Design review of the part built by this model. Coordinates are the model's own, in mm. A direction names the side the tool comes from. Round coordinates to 2 decimals unless told otherwise and drop trailing zeros. Order: outer loops, then holes, each group sorted by start corner. A loop starts at its lowest first (then second) coordinate and runs counter-clockwise, first axis right, second up. Notation, with made-up numbers: M 21,46 L 33,46 A27 ccw 33,68 Z; hole C 68,-40 d6. An arc over 180 degrees is marked long. Use a Markdown table: item, result. Add a question column.
(1) Take a section at C-C (z = -11). Write out the cut boundary in (x, y), then the cut area to 3 significant figures.
(2) Machinability: for faces 5 (the face through (2.36, 5.87, 21.9)), 6 (the face through (4.483, 2.532, -23.147)), 7 (the face through (2.4, 5.87, -21.86)), which of the approach directions +Z, -Z, +X, -X, +Y, -Y give a long, thin tool a straight path to every point of the face, cutting with its end or side? Answer none if there is none.
(3) The part is to be moulded in two halves that separate along Y. For faces 1 (the face through (0, 0, 6)), 2 (the face through (8, 5.5, 24)), 3 (the face through (10.55, 2.58, 18.9)), 4 (the face through (-7.83, 1.97, 6.53)), say which applies: released by +Y, released by -Y, zero draft, split by the parting line, or undercut.
(4) To check wall thickness, follow probe 1 along X at (y, z) = (2.75, -21.75); probe 2 along Z at (x, y) = (-5, 5); probe 3 along Z at (x, y) = (0, 0.95). State the ranges of each line that lie inside material, in increasing order. Write a range as from..to.
(5) For pin 1 (1.8 mm diameter, centred on x = -3.5, y = 2.75, fed in from +Z); pin 2 (1.5 mm diameter, centred on x = 0, z = -11, fed in from -Y); pin 3 (4 mm diameter, centred on x = -10, z = 2, fed in from +Y), all flat-tipped, find the tip position at first contact; note any pin that passes through.
(6) Take a section at A-A (x = 0). Write out the cut boundary in (y, z).
(7) Take a section at B-B (y = 4.5). Write out the cut boundary in (x, z), then the cut area to 3 significant figures.
(8) Take a section at D-D (z = 22). Write out the cut boundary in (x, y).
Autodesk Inventor part; units mm, degrees
ref_plane "YZ Plane" through (0, 0, 0) normal (1, 0, 0) x (0, 1, 0)
ref_plane "XZ Plane" through (0, 0, 0) normal (0, 1, 0) x (-1, 0, 0)
ref_plane "XY Plane" through (0, 0, 0) normal (0, 0, 1) x (1, 0, 0)
sketch "Sketch1" plane through (0, 0, 0) normal (0, 1, 0) x (-1, 0, 0)
  line L0 (15, 27) -> (-15, 27)
  line L1 (-15, 27) -> (-15, -27)
  line L2 (-15, -27) -> (15, -27)
  line L3 (15, -27) -> (15, 27)
  line L4 (0, 27) -> (0, -27) construction
  line L5 (15, 0) -> (-15, 0) construction
  point P0 (0, 0)
  point P1 (0, 0)
  point P2 (15, 0)
  dimension "d0" = 54
  dimension "d1" = 30
extrude "Extrusion1" add sketch "Sketch1" along normal blind 6.25
sketch "Sketch2" plane through (0, 6.25, 0) normal (0, 1, 0) x (1, 0, 0)
  circle A0 centre (0, 0) radius 11 construction
  line L0 (0, 0) -> (-15, 0) construction
  line L1 (-35.2782, 0) -> (23.3797, 0) construction
  line L2 (0, 37.8) -> (0, -37.8) construction
  line L3 (-15, -27) -> (15, -27)
  line L4 (15, -27) -> (15, 27)
  line L5 (15, 27) -> (-15, 27)
  line L6 (-15, 27) -> (-15, -27)
  line L7 (-15, 27) -> (-15, -27)
  point P0 (-11, 0)
  point P1 (-7.7782, -7.7782)
  point P2 (0, -11)
  point P3 (7.7782, -7.7782)
  point P4 (11, 0)
  point P5 (7.7782, 7.7782)
  point P6 (0, 11)
  point P7 (-7.7782, 7.7782)
  dimension "d7" = 22
  dimension "d8" = 360
hole "Hole1" at (-11, 6.25, 0) at (-7.7782, 6.25, -7.7782) at (0, 6.25, -11) at (7.7782, 6.25, -7.7782) at (11, 6.25, 0) at (7.7782, 6.25, 7.7782) at (0, 6.25, 11) at (-7.7782, 6.25, 7.7782) direction (0, -1, 0) diameter 2.5 end through all
sketch "Sketch3" plane through (0, 6.25, 0) normal (0, 1, 0) x (1, 0, 0)
  circle A0 centre (0, 0) radius 5.05
  dimension "d17" = 10.1
extrude "Extrusion2" cut sketch "Sketch3" against normal through all
sketch "Sketch6" plane through (-15, 0, 27) normal (0, 0, 1) x (1, 0, 0)
  line L0 (-10.3797, 2.75) -> (37.9037, 2.75) construction
  line L1 (0, 0) -> (30, 0) construction
  line L2 (0, 0) -> (0, 6.25)
  point P0 (15, 0)
  point P1 (4.5, 2.75)
  point P2 (11.5, 2.75)
  point P3 (18.5, 2.75)
  point P4 (25.5, 2.75)
  dimension "d33" = 2.75
  dimension "d34" = 4.5
  dimension "d37" = 7
hole "Hole3" at (-10.5, 2.75, 27) at (-3.5, 2.75, 27) at (3.5, 2.75, 27) at (10.5, 2.75, 27) direction (0, 0, -1) diameter 2.013 depth 7.6 tip angle 118
sketch "Sketch7" plane through (15, 0, -27) normal (0, 0, -1) x (-1, 0, 0)
  line L0 (-10.51, 2.75) -> (37.7733, 2.75) construction
  line L1 (0, 0) -> (29.8697, 0) construction
  line L2 (0, 0) -> (0, 3.7534)
  line L3 (0, 0) -> (30, 0)
  line L4 (0, 0) -> (0, 6.25)
  point P0 (15, 0)
  point P1 (15, 0)
  point P2 (4.5, 2.75)
  point P3 (11.5, 2.75)
  point P4 (18.5, 2.75)
  point P5 (25.5, 2.75)
  dimension "d53" = 2.75
  dimension "d54" = 4.5
  dimension "d55" = 7
hole "Hole4" at (10.5, 2.75, -27) at (-10.5, 2.75, -27) at (-3.5, 2.75, -27) at (3.5, 2.75, -27) direction (0, 0, 1) diameter 2.013 depth 7.6 tip angle 118
sketch "Sketch8" plane through (0, 6.25, 0) normal (0, 1, 0) x (1, 0, 0)
  line L0 (0, 38.85) -> (0, -39.55) construction
  line L1 (-15, -27) -> (15, -27)
  line L2 (15, 27) -> (-15, 27)
  line L3 (-1.5, -27) -> (-15, -27)
  line L4 (-15, -27) -> (-15, -21)
  line L5 (-15, -21) -> (-1.5, -21)
  line L6 (1.5, -27) -> (15, -27)
  line L7 (15, -27) -> (15, -21)
  line L8 (15, -21) -> (1.5, -21)
  line L9 (15, -27) -> (15, 27)
  line L10 (-15, 27) -> (-15, -27)
  line L11 (-1.5, -21) -> (-1.5, -27)
  line L12 (-15, -27) -> (15, -27)
  line L13 (1.5, -21) -> (1.5, -27)
  line L14 (-15, 0) -> (15, 0) construction
  line L15 (-1.5, 27) -> (-15, 27)
  line L16 (-15, 27) -> (-15, 21)
  line L17 (-15, 21) -> (-1.5, 21)
  line L18 (1.5, 27) -> (15, 27)
  line L19 (15, 27) -> (15, 21)
  line L20 (15, 21) -> (1.5, 21)
  line L21 (-1.5, 21) -> (-1.5, 27)
  line L22 (1.5, 21) -> (1.5, 27)
  line L23 (-21.8515, -25) -> (23.2072, -25) construction
  point P0 (0, 0)
  dimension "d80" = 6
  dimension "d81" = 3
  dimension "d82" = 13.5
  dimension "d86" = 2
extrude "Extrusion6" cut sketch "Sketch8" against normal blind 0.75 contours L4 L5 L11 L1 | L13 L8 L7 L1 | L10 L2 L21 L17 | L20 L22 L2 L9
fillet "Fillet1" radius 3 4 edges at (1.5, 5.875, 21) (-1.5, 5.875, 21) (1.5, 5.875, -21) (-1.5, 5.875, -21)
sketch "Sketch11" plane through (0, 6.25, 0) normal (0, 1, 0) x (1, 0, 0)
  line L0 (-13.5, -19.5) -> (13.5, -19.5)
  line L1 (13.5, -19.5) -> (13.5, 19.5)
  line L2 (13.5, 19.5) -> (-13.5, 19.5)
  line L3 (-13.5, 19.5) -> (-13.5, -19.5)
  line L4 (-15, 21) -> (-15, -21)
  line L5 (15, -21) -> (15, 21)
  line L6 (-1.5, -27) -> (-15, -27)
  line L7 (-15, 27) -> (-1.5, 27)
  point P0 (0, 0)
  dimension "d87" = 7.5
  dimension "d88" = 7.5
  dimension "d91" = 1.5
  dimension "d92" = 1.5
extrude "Extrusion7" cut sketch "Sketch11" against normal blind 2.25
fillet "Fillet2" radius 1.5 4 edges at (-13.5, 5.125, 19.5) (13.5, 5.125, 19.5) (13.5, 5.125, -19.5) (-13.5, 5.125, -19.5)
equation "\"d0\" = u_internal_width + 2 * u_side_trace_depth"
equation "\"d1\" = u_internal_depth"
equation "\"d3\" = plate_thickness"
equation "\"d7\" = d9"
equation "\"d18\" = plate_thickness"
equation "\"d33\" = hole_2_bottom"
equation "\"d53\" = hole_2_bottom"
equation "\"d83\" = plate_thickness - border_thickness"
equation "\"plate_thickness\" = 6.25"
equation "\"d9\" = 22"
equation "\"tol\" = 0.1"
equation "\"u_internal_width\" = 52"
equation "\"u_internal_depth\" = 30"
equation "\"u_side_trace_depth\" = 1"
equation "\"border_thickness\" = 5.5"
equation "\"hole_2_bottom\" = 0.5 * border_thickness"
properties part number "new_base_u106_long_newbearing" material "Aluminum 2014-T4"
Verdict:
| question | item | result |
|---|---|---|
| 1 | outline | M -15,0 L -1.25,0 L -1.25,4 L -13.5,4 L -13.5,6.25 L -15,6.25 Z; M 1.25,0 L 15,0 L 15,6.25 L 13.5,6.25 L 13.5,4 L 1.25,4 Z |
| 1 | area | 117 mm^2 |
| 2 | face 5 | +Z, +X, +Y |
| 2 | face 6 | -Z |
| 2 | face 7 | -Z, +X, +Y |
| 3 | face 1 | released by -Y |
| 3 | face 2 | released by +Y |
| 3 | face 3 | undercut |
| 3 | face 4 | zero draft |
| 4 | probe 1 | x = -15..-11.51, -9.49..-4.51, -2.49..2.49, 4.51..9.49, 11.51..15 |
| 4 | probe 2 | z = -27..-19.5, 19.5..27 |
| 4 | probe 3 | z = -27..-12.25, -9.75..-5.05, 5.05..9.75, 12.25..27 |
| 5 | pin 1 | stops at z = 19.34 |
| 5 | pin 2 | passes through |
| 5 | pin 3 | stops at y = 4 |
| 6 | outline | M 0,-27 L 6.25,-27 L 6.25,-19.5 L 4,-19.5 L 4,-12.25 L 0,-12.25 Z; M 0,-9.75 L 4,-9.75 L 4,-5.05 L 0,-5.05 Z; M 0,5.05 L 4,5.05 L 4,9.75 L 0,9.75 Z; M 0,12.25 L 4,12.25 L 4,19.5 L 6.25,19.5 L 6.25,27 L 0,27 Z |
| 7 | outline | M -15,-27 L 15,-27 L 15,27 L -15,27 Z; hole M -13.5,-18 A1.5 ccw -12,-19.5 L 12,-19.5 A1.5 ccw 13.5,-18 L 13.5,18 A1.5 ccw 12,19.5 L -12,19.5 A1.5 ccw -13.5,18 Z |
| 7 | area | 569 mm^2 |
| 8 | outline | M -15,0 L 15,0 L 15,5.5 L 2.26,5.5 L 2.26,6.25 L -2.26,6.25 L -2.26,5.5 L -15,5.5 Z; hole C -10.5,2.75 d2.01; hole C -3.5,2.75 d2.01; hole C 3.5,2.75 d2.01; hole C 10.5,2.75 d2.01 |
